Check sheet for the modelled part. Datum: model origin and axes. Units: mm. Face numbers are marked on the shaded views. A direction names the side the tool comes from. Coordinates: 2 decimals unless noted, no trailing zeros. Write each loop counter-clockwise with the first axis right and the second up, starting at its lowest first coordinate (ties: lowest second). Pieces come first, ordered by that corner, then holes. Notation, with made-up numbers: (20, -8.5) -> (39, -8.5) arc R19 ccw to (39, 0.5) -> close; hole circle Ø4 at (5.5, -9). An arc over 180 degrees is marked (long way). Put each result on its own line as item: value.
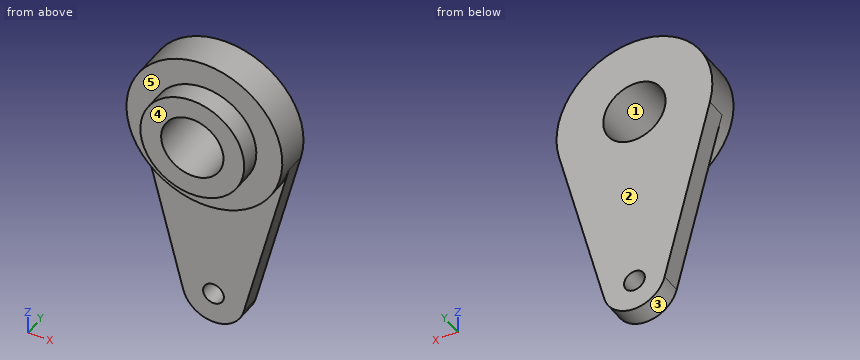
```python
from build123d import *

# Parameters (mm, degrees)
SKETCH_1_R          = 5
EXTRUDE_1_DEPTH     = 2
SKETCH_2_R          = 7.5
EXTRUDE_2_DEPTH     = 1.5
SKETCH_3_R          = 1
EXTRUDE_3_DEPTH     = 2
SKETCH_4_R          = 3
CUT_EXTRUDE_1_DEPTH = 23.967368156


with BuildPart() as part:
    # 草图1 → 凸台-拉伸1 (new body)
    with BuildSketch(Plane(origin=(0, 0, 0), x_dir=(1, 0, 0), z_dir=(0, 1, 0))):
        with Locations(Location((0, 0, 0), (0, 0, 270))):
            Circle(SKETCH_1_R)
    extrude(amount=EXTRUDE_1_DEPTH)

    # 草图2 → 凸台-拉伸2 (add)
    with BuildSketch(Plane(origin=(0, 2, 0), x_dir=(1, 0, 0), z_dir=(0, 1, 0))):
        with Locations(Location((0, 0, 0), (0, 0, 270))):
            Circle(SKETCH_2_R)
    extrude(amount=EXTRUDE_2_DEPTH)

    # 草图3 → 凸台-拉伸3 (add)
    with BuildSketch(Plane(origin=(0, 3.5, 0), x_dir=(1, 0, 0), z_dir=(0, 1, 0))):
        with BuildLine():
            Line((-2.90473751, 18.75), (-7.261843774, 1.875))
            ThreePointArc((-7.261843774, 1.875), (0, -7.5), (7.261843774, 1.875))
            Line((7.261843774, 1.875), (2.90473751, 18.75))
            ThreePointArc((2.90473751, 18.75), (0, 21), (-2.90473751, 18.75))
        make_face()
        with Locations(Location((0, 18, 0), (0, 0, 270))):
            Circle(SKETCH_3_R, mode=Mode.SUBTRACT)
    extrude(amount=EXTRUDE_3_DEPTH)

    # 草图4 → 切除-拉伸1 (cut, through all)
    with BuildSketch(Plane.XZ):
        with Locations(Location((0, 0, 0), (0, 0, 270))):
            Circle(SKETCH_4_R)
    extrude(amount=-CUT_EXTRUDE_1_DEPTH, mode=Mode.SUBTRACT)


solid = part.part
```
Q1. Tool access check on the marked faces 4 and 5. Record the directions out of +Z, -Z, +X, -X, +Y, -Y that give a thin tool (end or side, any length) a straight path to the whole face; none if there is none.
Recorded:
face 4: +Z, -Z, +X, -X, -Y
face 5: -Y
Q2. Mould release check, pull along Z, two halves, no side actions. Record for the marked faces 1, 2 and 3: released by +Z, released by -Z, zero draft, split by the parting line, or undercut.
Recorded:
face 1: undercut
face 2: zero draft
face 3: released by -Z
Q3. Material ranges on line 1 along X through (y, z) = (1.3, 0); line 2 along X through (y, z) = (3.35, 0); line 3 along Y through (x, z) = (4.25, -5.5), recorded low to high.
Recorded:
line 1: x = -5 to -3, 3 to 5
line 2: x = -7.5 to -3, 3 to 7.5
line 3: y = 2 to 5.5
Q4. Cross-section at C-C (y = 0.9). Record the cut outline in (x, z), plus the area to 3 significant figures.
Recorded:
outline: circle Ø10 at (0, 0); hole circle Ø6 at (0, 0)
area: 50.3 mm2
Q5. Depth check by flat-ended pin: P1, Ø6, axis at x = 0.5, z = 2, coming from the +Y side; P2, Ø4.5, axis at x = 0, z = -15.5, coming from the -Y side; P3, Ø1, axis at y = 4.5, z = -3, coming from the -X side; P4, Ø1.5, axis at y = 4, z = -14, coming from the +X side. Enter the tip coordinate at first touch or a pass-through.
Recorded:
P1: stops at y = 5.5
P2: stops at y = 3.5
P3: stops at x = -7.1
P4: stops at x = 4.32
Q6. Cross-section at D-D (x = -1.5). Record the cut outline in (y, z).
Recorded:
outline: (0, -4.77) -> (2, -4.77) -> (2, -7.35) -> (3.5, -7.35) -> (3.5, -20.6) -> (5.5, -20.6) -> (5.5, -2.6) -> (0, -2.6) -> close; (0, 2.6) -> (5.5, 2.6) -> (5.5, 7.35) -> (2, 7.35) -> (2, 4.77) -> (0, 4.77) -> close
Q7. Cross-section at B-B (z = 0). Record the cut outline in (x, y), plus the area to 3 significant figures.
Recorded:
outline: (-7.5, 2) -> (-5, 2) -> (-5, 0) -> (-3, 0) -> (-3, 5.5) -> (-7.5, 5.5) -> close; (3, 0) -> (5, 0) -> (5, 2) -> (7.5, 2) -> (7.5, 5.5) -> (3, 5.5) -> close
area: 39.5 mm2
Q8. Cross-section at A-A (x = 0). Record the cut outline in (y, z), plus the area to 3 significant figures.
Recorded:
outline: (0, -5) -> (2, -5) -> (2, -7.5) -> (3.5, -7.5) -> (3.5, -17) -> (5.5, -17) -> (5.5, -3) -> (0, -3) -> close; (0, 3) -> (5.5, 3) -> (5.5, 7.5) -> (2, 7.5) -> (2, 5) -> (0, 5) -> close; (3.5, -21) -> (5.5, -21) -> (5.5, -19) -> (3.5, -19) -> close
area: 62.5 mm2
